Model file for the job. Use its own axes, mm. Round coordinates to 2 decimals unless told otherwise and drop trailing zeros. Loops run counter-clockwise (first coordinate to the right, second up) from the corner with the lowest first, then second, coordinate; pieces in that order, holes last. Notation, with made-up numbers: (21, -30.5) - (56, -30.5) arc R25 cw to (56, 7.5) - close; hole circle Ø1 at (33.25, -10). An arc over 180 degrees is marked (long way). Use one line per item in the form item = value.
from build123d import *

# Parameters (mm, degrees)
SKETCH1_R           = 73.029292346
BOSS_EXTRUDE1_DEPTH = 3.175
SKETCH8_R           = 6.35
CUT_EXTRUDE3_DEPTH  = 16.256
SKETCH10_R          = 6.731
CUT_EXTRUDE4_DEPTH  = 25.4
SKETCH11_R          = 3.571875
CUT_EXTRUDE5_DEPTH  = 254


with BuildPart() as part:
    # Sketch1 → Boss-Extrude1 (new body)
    with BuildSketch(Plane(origin=(0, 0, 0), x_dir=(1, 0, 0), z_dir=(0, 1, 0))):
        with Locations(Location((0, 0, 0), (0, 0, 270))):
            Circle(SKETCH1_R)
    extrude(amount=BOSS_EXTRUDE1_DEPTH)

    # Sketch8 → Cut-Extrude3 (cut)
    with BuildSketch(Plane(origin=(0, 3.175, 0), x_dir=(1, 0, 0), z_dir=(0, 1, 0))):
        with Locations(Location((0, 0, 0), (0, 0, 270))):
            Circle(SKETCH8_R)
    extrude(amount=-CUT_EXTRUDE3_DEPTH, mode=Mode.SUBTRACT)

    # Sketch10 → Cut-Extrude4 (cut)
    with BuildSketch(Plane(origin=(0, 3.175, 0), x_dir=(1, 0, 0), z_dir=(0, 1, 0))):
        with Locations(Location((-63.5, 0, 0), (0, 0, 270))):
            Circle(SKETCH10_R)
        with Locations(Location((63.5, 0, 0), (0, 0, 270))):
            Circle(SKETCH10_R)
    extrude(amount=-CUT_EXTRUDE4_DEPTH, mode=Mode.SUBTRACT)

    # Sketch11 → Cut-Extrude5 (cut)
    with BuildSketch(Plane(origin=(0, 3.175, 0), x_dir=(1, 0, 0), z_dir=(0, 1, 0))):
        with Locations(Location((-52.128653384, -23.424901204, 0), (0, 0, 270))):
            Circle(SKETCH11_R)
        with Locations(Location((52.128653384, 23.424901204, 0), (0, 0, 270))):
            Circle(SKETCH11_R)
    extrude(amount=-CUT_EXTRUDE5_DEPTH, mode=Mode.SUBTRACT)


solid = part.part
1. Pull direction X, two halves, no side cores. Call faces 1 (the cylindrical face through (21.936, 1.565, 69.657)), 2 (the flat face through (-15, 0, -1)), 3 (the cylindrical face through (55.67, 1.61, -23.89)): +X half, -X half, draft (parallel to the pull), parting line (faces both ways), or undercut.
Geometry check:
face_1 = parting line
face_2 = draft
face_3 = undercut
2. Wall check: probe 1 along X at (y, z) = (1.8, 0); probe 2 along Z at (x, y) = (57.5, 3); probe 3 along X at (y, z) = (2.75, -1.5). Give the ranges that are in metal, low to high.
Geometry check:
probe_1 = -73.03 to -70.23, -56.77 to -6.35, 6.35 to 56.77, 70.23 to 73.03
probe_2 = -45.02 to -3.05, 3.05 to 45.02
probe_3 = -73.01 to -70.06, -56.94 to -6.17, 6.17 to 56.94, 70.06 to 73.01
3. Cut at A-A, the plane x = 0. Give the cut face in (y, z) (3 decimals), plus the area to 3 significant figures.
Geometry check:
outline = (0, -73.029) - (3.175, -73.029) - (3.175, -6.35) - (0, -6.35) - close; (0, 6.35) - (3.175, 6.35) - (3.175, 73.029) - (0, 73.029) - close
area = 423 mm^2
4. Flat gauge pin, fed straight in: pin 1 (12 mm diameter, centred on x = -63.5, z = 0, fed in from -Y). Where does the tip first touch, or does it go through?
Geometry check:
pin_1 = through
5. Cut at B-B, the plane z = 0. Give the cut face in (x, y) (3 decimals).
Geometry check:
outline = (-73.029, 0) - (-70.231, 0) - (-70.231, 3.175) - (-73.029, 3.175) - close; (-56.769, 0) - (-6.35, 0) - (-6.35, 3.175) - (-56.769, 3.175) - close; (6.35, 0) - (56.769, 0) - (56.769, 3.175) - (6.35, 3.175) - close; (70.231, 0) - (73.029, 0) - (73.029, 3.175) - (70.231, 3.175) - close
6. Cut at D-D, the plane y = 2.65. Give the cut face in (x, z), plus the area to 3 significant figures.
Geometry check:
outline = circle Ø146.06 at (0, 0); hole circle Ø13.46 at (-63.5, 0); hole circle Ø7.14 at (-52.13, 23.42); hole circle Ø12.7 at (0, 0); hole circle Ø7.14 at (52.13, -23.42); hole circle Ø13.46 at (63.5, 0)
area = 16,300 mm^2
7. Cut at C-C, the plane z = 25. Give the cut face in (x, y) (3 decimals).
Geometry check:
outline = (-68.617, 0) - (-55.334, 0) - (-55.334, 3.175) - (-68.617, 3.175) - close; (-48.923, 0) - (68.617, 0) - (68.617, 3.175) - (-48.923, 3.175) - close
